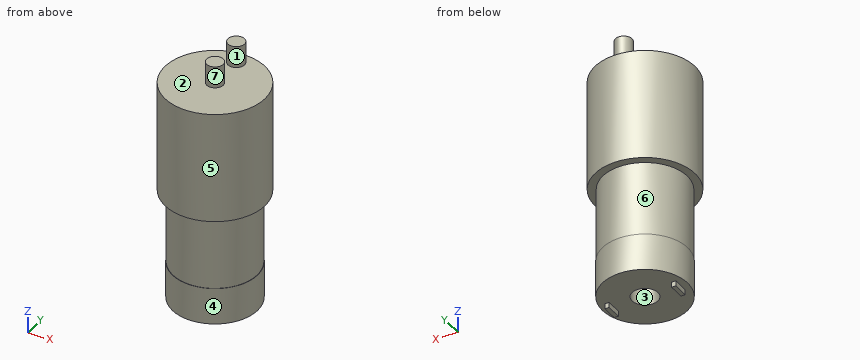
from build123d import *

# Parameters (mm, degrees)
F0_W      = 4.18402
F0_H      = 30
F2_R      = 13.5
F3_DEPTH  = 30
F4_R      = 11.5
F5_DEPTH  = 9.9
F6_W      = 1.150094
F6_H      = 4.307738
F7_DEPTH  = 1.4
F6_R      = 3.498999
F8_DEPTH  = 34.8
F9_R      = 2.25
F10_DEPTH = 5.85


with BuildPart() as f1:
    # F0 (on Right) → F1 (revolve)
    with BuildSketch(Plane.YZ):
        with Locations((-9.298615, 15)):
            Rectangle(F0_W, F0_H)
    revolve(axis=Axis((0, 0, 13.057403), (0, 0, -1)))

    # F2 (on face) → F3 (join)
    with BuildSketch(Plane.XY.offset(30)):
        Circle(F2_R)
    extrude(amount=F3_DEPTH)

    # F4 (on face) → F5 (join)
    with BuildSketch(Plane(origin=(0, 0, 0), x_dir=(1, 0, 0), z_dir=(0, 0, -1))):
        Circle(F4_R)
    extrude(amount=-F5_DEPTH)

    # F6 (on face) → F7 (join)
    with BuildSketch(Plane(origin=(0, 0, 0), x_dir=(1, 0, 0), z_dir=(0, 0, -1))):
        with Locations((-9, 0)):
            Rectangle(F6_W, F6_H)
        with Locations((9, 0)):
            Rectangle(F6_W, F6_H)
    extrude(amount=F7_DEPTH)

    # F6 (on face) → F8 (cut)
    with BuildSketch(Plane(origin=(0, 0, 0), x_dir=(1, 0, 0), z_dir=(0, 0, -1))):
        Circle(F6_R)
    extrude(amount=-F8_DEPTH, mode=Mode.SUBTRACT)

    # F9 (on face) → F10 (join)
    with BuildSketch(Plane.XY.offset(60)):
        Circle(F9_R)
        with Locations((0, 9.85)):
            Circle(F9_R)
    extrude(amount=F10_DEPTH)


solid = f1.part
Can you work these out from the model? Positions are in its coordinate system, mm. Face numbers are marked on the shaded views. A direction names the side the tool comes from. Coordinates: 2 decimals unless noted, no trailing zeros. Loops run counter-clockwise (first coordinate to the right, second up) from the corner with the lowest first, then second, coordinate; pieces in that order, holes last. Notation, with made-up numbers: M 85,70.25 L 143,70.25 A16 cw 143,87.25 Z; hole C 46,11 d2. An arc over 180 degrees is marked long. Answer as CSV lines item,"result". Start each with the question number.
1. For pin 1 Ø1 at (x, z) = (2.5, 37) entering from -Y; pin 2 Ø1 at (y, z) = (2, 48.5) entering from +X; pin 3 Ø1 at (x, z) = (-9, 41.5) entering from +Y, each with a flat end and sliding along its axis, tell me the tip position at first contact or that it passes through.
2. For the marked faces 4, 5, 6 and 7, which set-ups out of +Z, -Z, +X, -X, +Y, -Y let a thin tool reach every point of the face, with its end or its side?
3. Thinking about a two-plate mould opening in X: for the marked faces 1, 2 and 3, which applies, +X half, -X half, draft (parallel to the pull), parting line (faces both ways), or undercut?
4. Suppose I cut it at A-A, the plane x = -4.5. List the corners of the cut face in (y, z) for me.
5. Suppose I cut it at C-C, the plane y = 4.25. List the corners of the cut face in (x, z) for me, plus the area to 3 significant figures.
6. Suppose I cut it at B-B, the plane z = 12. List the corners of the cut face in (x, y) for me.
7. If I drill on probe 1 along Y at (x, z) = (0, 25.5); probe 2 along Z at (x, y) = (4.25, -1.75); probe 3 along X at (y, z) = (0, 5.25), over which ranges is the centre line in solid material (lowest first)? Write a range as [from, to].
Output:
1,pin 1,"stops at y = -13.35"
1,pin 2,"stops at x = 13.42"
1,pin 3,"stops at y = 10.49"
2,face 4,"-Z"
2,face 5,"+Z, -Z"
2,face 6,"none"
2,face 7,"+Z"
3,face 1,"parting line"
3,face 2,"draft"
3,face 3,"undercut"
4,outline,"M -12.73,30 L -10.46,30 L -10.46,9.9 L -10.58,9.9 L -10.58,0 L 10.58,0 L 10.58,9.9 L 10.46,9.9 L 10.46,30 L 12.73,30 L 12.73,60 L -12.73,60 Z; hole M -5.63,9.9 L 5.63,9.9 L 5.63,30 L -5.63,30 Z"
5,outline,"M -12.81,30 L -10.57,30 L -10.57,9.9 L -10.69,9.9 L -10.69,0 L 10.69,0 L 10.69,9.9 L 10.57,9.9 L 10.57,30 L 12.81,30 L 12.81,60 L -12.81,60 Z; hole M -5.82,9.9 L 5.82,9.9 L 5.82,30 L -5.82,30 Z"
5,area,"1,170 mm^2"
6,outline,"C 0,0 d22.78; hole C 0,0 d14.41"
7,probe 1,"y = [-11.39, -7.21], [7.21, 11.39]"
7,probe 2,"z = [0, 9.9], [30, 60]"
7,probe 3,"x = [-11.5, -3.5], [3.5, 11.5]"
